Autodesk Inventor part; units mm, degrees
ref_plane "YZ Plane" through (0, 0, 0) normal (1, 0, 0) x (0, 1, 0)
ref_plane "XZ Plane" through (0, 0, 0) normal (0, 1, 0) x (-1, 0, 0)
ref_plane "XY Plane" through (0, 0, 0) normal (0, 0, 1) x (1, 0, 0)
sketch "Sketch1" plane through (0, 0, 0) normal (0, 1, 0) x (-1, 0, 0)
  circle A0 centre (0, 0) radius 2.5
  dimension "d0" = 5
extrude "Extrusion1" add sketch "Sketch1" along normal blind 12
sketch "Sketch5" plane through (0, 12, 0) normal (0, 1, 0) x (1, 0, 0)
  circle A0 centre (0, 0) radius 2.5
  circle A1 centre (0, 0) radius 4
  dimension "d20" = 8
extrude "Extrusion5" add sketch "Sketch5" along normal blind 300 contours A0 | A1
sketch "Sketch6" plane through (0, 312, 0) normal (0, 1, 0) x (1, 0, 0)
  circle A0 centre (0, 0) radius 4
  circle A1 centre (0, 0) radius 2.5
  dimension "d23" = 5
extrude "Extrusion6" add sketch "Sketch6" along normal blind 5 contours A1
thread "Thread2"
thread "Thread3"
properties material "Steel"
The model under review builds one solid part; all positions refer to its coordinate system, in mm. A direction names the side the tool comes from. Round coordinates to 2 decimals unless told otherwise and drop trailing zeros. Order: outer loops, then holes, each group sorted by start corner. A loop starts at its lowest first (then second) coordinate and runs counter-clockwise, first axis right, second up.
Item 1: Add section B-B, the plane z = 0. State the section outline as (x, y) points, and give its area (4 significant figures).
Working result:
outline: (-4, 12) - (-2.5, 12) - (-2.5, 0) - (2.5, 0) - (2.5, 12) - (4, 12) - (4, 312) - (2.5, 312) - (2.5, 317) - (-2.5, 317) - (-2.5, 312) - (-4, 312) - close
area: 2,485 mm2
Item 2: Add section C-C, the plane y = 50. State the section outline as (x, z) points, and give its area (3 significant figures).
Working result:
outline: circle Ø8 at (0, 0)
area: 50.3 mm2
Item 3: For pin 1 (1.5 mm diameter, centred on y = 94, z = 1, fed in from -X); pin 2 (1.5 mm diameter, centred on x = -2.5, y = 109, fed in from -Z), all flat-tipped, find the tip position at first contact; note any pin that passes through.
Working result:
pin 1: stops at x = -3.99
pin 2: stops at z = -3.6
Item 4: To check wall thickness, follow probe 1 along Z at (x, y) = (0.25, 257); probe 2 along Y at (x, z) = (-3, 0.25). State the ranges of each line that lie inside material, in increasing order.
Working result:
probe 1: z = -3.99 to 3.99
probe 2: y = 12 to 312
Item 5: Machinability: for faces 1 (the cylindrical face through (-0.867, 159.9, -3.905)), 2 (the cylindrical face through (-0.54, 314.46, -2.44)), 3 (the cylindrical face through (0.54, 5.92, 2.44)), which of the approach directions +Z, -Z, +X, -X, +Y, -Y give a long, thin tool a straight path to every point of the face, cutting with its end or side? Answer none if there is none.
Working result:
face 1: +Y, -Y
face 2: +Y
face 3: -Y
Item 6: Add section A-A, the plane x = 0. State the section outline as (y, z) points, and give its area (4 significant figures).
Working result:
outline: (0, -2.5) - (12, -2.5) - (12, -4) - (312, -4) - (312, -2.5) - (317, -2.5) - (317, 2.5) - (312, 2.5) - (312, 4) - (12, 4) - (12, 2.5) - (0, 2.5) - close
area: 2,485 mm2
